from build123d import *

# Parameters (mm, degrees)
F1_DEPTH = 23
F2_COUNT = 12
F0_R     = 8.9323365914
F3_DEPTH = 29.2


with BuildPart() as f1:
    # F0 (on Front) → F1 (new body)
    with BuildSketch(Plane.XZ):
        with BuildLine():
            ThreePointArc((-1.430105941, 37.8043599743), (2.9480264381, 38.3709128978), (7.3598275006, 38.21268291))
            ThreePointArc((7.3598275006, 38.21268291), (7.1059115447, 40.6764495808), (6.4814269965, 43.0732471463))
            ThreePointArc((6.4814269965, 43.0732471463), (5.2761037826, 45.5878183542), (3.6249864327, 47.8349685287))
            ThreePointArc((3.6249864327, 47.8349685287), (2.2938527312, 48.2892841606), (1.0334071525, 47.6651074485))
            ThreePointArc((1.0334071525, 47.6651074485), (-0.310272704, 45.2216678947), (-1.1770668058, 42.5712829425))
            ThreePointArc((-1.1770668058, 42.5712829425), (-1.4791386758, 40.1971401747), (-1.430105941, 37.8043599743))
        make_face()
        with BuildLine():
            ThreePointArc((-1.430105941, 37.8043599743), (-12.6935408321, -9.348025826), (31.0549458343, 11.5393475513))
            ThreePointArc((31.0549458343, 11.5393475513), (24.2756583786, 29.3783879684), (7.3598275006, 38.21268291))
            ThreePointArc((7.3598275006, 38.21268291), (2.9480264381, 38.3709128978), (-1.430105941, 37.8043599743))
        make_face()
        Polygon((0.3031889381, 26.7559829898), (15.426810236, 22.5175925953), (19.3180671322, 7.3009571569), (8.0857027305, -3.6772878871), (-7.0379185674, 0.5611025073), (-10.9291754636, 15.7777379458), align=None, mode=Mode.SUBTRACT)
    extrude(amount=F1_DEPTH)

    # F2: F1 ×12 about axis
    f2_axis = Axis((4.1944458343, 0, 11.5393475513), (0, 1, 0))


with BuildPart() as f1_1:
    add(f1.part)
    for i in range(1, F2_COUNT):
        add(f1.part.rotate(f2_axis, i * 360 / F2_COUNT))

    # F0 (on Front) → F3 (join)
    with BuildSketch(Plane.XZ):
        Polygon((19.3180671322, 7.3009571569), (15.426810236, 22.5175925953), (0.3031889381, 26.7559829898), (-10.9291754636, 15.7777379458), (-7.0379185674, 0.5611025073), (8.0857027305, -3.6772878871), align=None)
        with Locations((4.1944458343, 11.5393475513)):
            Circle(F0_R, mode=Mode.SUBTRACT)
    extrude(amount=F3_DEPTH)


solid = f1_1.part
Work out the finished part from the listing and answer in its coordinate system (mm). A direction names the side the tool comes from. Give positions to 0.01 mm unless a question says otherwise; leave off trailing zeros. Loops run counter-clockwise (first coordinate to the right, second up) from the corner with the lowest first, then second, coordinate; pieces in that order, holes last. Notation, with made-up numbers: (11, 23) -> (39, 23) arc R27 cw to (39, 50) -> close; hole circle Ø5 at (80.25, 28.25). An arc over 180 degrees is marked (long way). Use a Markdown table: item, result. Add a question column.
1. Section A-A on x = -3 is taken. Determine the outline of the cut face in (y, z).
2. Flat-ended cylindrical pins translate along their axes: pin 1 Ø8 at (y, z) = (-18, -15.5) entering from -X; pin 2 Ø6 at (y, z) = (-19.5, 18.5) entering from +X; pin 3 Ø12 at (x, y) = (-23.5, -24.5) entering from +Z. Find the tip coordinate at first contact, or state that the pin passes through.
3. Find the intervals of material crossed by probe 1 along Z at (x, y) = (31, -12.25); probe 2 along Y at (x, z) = (11.5, -10.5); probe 3 along X at (y, z) = (-6.5, 40.5), in increasing order.
4. Section C-C on z = -1 is taken. Determine the outline of the cut face in (x, y), and give its area (3 significant figures).
5. Determine the mould class of faces 1 (the cylindrical face through (22.31, -11.34, 31.37)), 2 (the cylindrical face through (3.093, -11.339, -22.476)), 3 (the cylindrical face through (2.31, -11.34, 48.29)), 4 (the cylindrical face through (21.27, -11.34, 35.28)) for opening direction X: released by +X, released by -X, zero draft, split by the parting line, or undercut.
6. Section B-B on y = -26.5 is taken. Determine the outline of the cut face in (x, z).
7. For faces 5 (the flat face through (0.42, -26.06, -1.53)), 6 (the cylindrical face through (-19.551, -11.339, 28.618)), 7 (the cylindrical face through (38.21, -11.34, 10.44)), 8 (the cylindrical face through (-13.924, -11.339, -8.29)), determine the directions among +Z, -Z, +X, -X, +Y, -Y from which every point of the face is accessible in a straight line to the end or side of a thin tool.
Results below:
| question | item | result |
|---|---|---|
| 1 | outline | (-29.2, -0.57) -> (-23, -0.57) -> (-23, -14.34) -> (0, -14.34) -> (0, 6.25) -> (-29.2, 6.25) -> close; (-29.2, 16.83) -> (0, 16.83) -> (0, 37.42) -> (-23, 37.42) -> (-23, 23.53) -> (-29.2, 23.53) -> close |
| 2 | pin 1 | stops at x = -13.77 |
| 2 | pin 2 | stops at x = 39 |
| 2 | pin 3 | stops at z = 29.5 |
| 3 | probe 1 | z = -6.3 to 2.64, 8.38 to 17.21, 23.69 to 32.27 |
| 3 | probe 2 | y = -23 to 0 |
| 3 | probe 3 | x = -16.64 to -10.24, -1.46 to 7.14, 14.55 to 22.16 |
| 4 | outline | (-23.05, -23) -> (-1.47, -23) -> (-1.47, -29.2) -> (10.82, -29.2) -> (10.82, -23) -> (35.31, -23) -> (35.31, 0) -> (-23.05, 0) -> close |
| 4 | area | 1,420 mm^2 |
| 5 | face 1 | undercut |
| 5 | face 2 | undercut |
| 5 | face 3 | split by the parting line |
| 5 | face 4 | released by +X |
| 6 | outline | (-10.93, 15.78) -> (-7.04, 0.56) -> (8.09, -3.68) -> (19.32, 7.3) -> (15.43, 22.52) -> (0.3, 26.76) -> close; hole circle Ø17.86 at (4.19, 11.54) |
| 7 | face 5 | -Z, -X, -Y |
| 7 | face 6 | +Z, +Y, -Y |
| 7 | face 7 | +X, +Y, -Y |
| 7 | face 8 | +Y, -Y |
